```python
from build123d import *

# Parameters (mm, degrees)
F0_W     = 41.710345
F0_H     = 19.551726
F0_W_2   = 8.255173
F0_H_2   = 5.21379
F0_W_3   = 9.55862
F0_H_3   = 4.779309
F1_DEPTH = 25
F2_R     = 1.5
F3_R     = 0.55
F4_R     = 1
F5_SIZE  = 2


with BuildPart() as f1:
    # F0 (on Top) → F1 (new body)
    with BuildSketch(Plane.XY):
        with Locations((-29.001724, 36.931037)):
            Rectangle(F0_W, F0_H)
        with Locations((-38.343103, 34.975864)):
            Rectangle(F0_W_2, F0_H_2, mode=Mode.SUBTRACT)
        with Locations((-20.746552, 37.799999)):
            Rectangle(F0_W_3, F0_H_3, mode=Mode.SUBTRACT)
    extrude(amount=-F1_DEPTH)

    # F2
    f2_edges = [f1.edges().sort_by_distance(p)[0] for p in [
        (-42.47069, 37.582759, -12.5),
        (-34.215517, 37.582759, -12.5),
        (-42.47069, 32.368969, -12.5),
        (-34.215517, 32.368969, -12.5),
        (-25.525862, 40.189654, -12.5),
    ]]
    fillet(f2_edges, radius=F2_R)

    # F3
    f3_edges = [f1.edges().sort_by_distance(p)[0] for p in [
        (-15.967242, 40.189654, -12.5),
        (-25.525862, 35.410345, -12.5),
        (-15.967242, 35.410345, -12.5),
    ]]
    fillet(f3_edges, radius=F3_R)

    # F4
    f4_edges = [f1.edges().sort_by_distance(p)[0] for p in [
        (-38.343104, 37.582759, 0),
    ]]
    fillet(f4_edges, radius=F4_R)

    # F5
    f5_edges = [f1.edges().sort_by_distance(p)[0] for p in [
        (-20.271552, 40.189654, 0),
    ]]
    chamfer(f5_edges, length=F5_SIZE)


solid = f1.part
```
Source: CAD feature listing. Evaluate the final solid. Frame: model axes, mm. A direction names the side the tool comes from. Round coordinates to 2 decimals unless told otherwise and drop trailing zeros. Loops run counter-clockwise (first coordinate to the right, second up) from the corner with the lowest first, then second, coordinate; pieces in that order, holes last. Notation, with made-up numbers: M 30,3 L 42,3 A10 ccw 42,16 Z; hole C 43,28.25 d5. An arc over 180 degrees is marked long. Use a Markdown table: item, result. Add a question column.
1. Ray query, line 1 along Y through (x, z) = (-19, -10.5); line 2 along X through (y, z) = (35.75, -21.5); line 3 along X through (y, z) = (35.5, -21.5). Return the intervals inside material, ascending. Write a range as [from, to].
2. Cut plane A-A, the plane z = -18.75. Output: boundary loops of the cut face in (x, y), and give its area (3 significant figures).
3. Pull-direction query (Y, two-part tool) for faces 1 (the flat face through (-29, 46.707, -12)), 2 (the flat face through (-8.147, 37, -12)), 3 (the flat face through (-15.967, 38, -13)); classes: +Y half, -Y half, draft (parallel to the pull), parting line (faces both ways), or undercut.
4. Set-up query: faces 4 (the flat face through (-34.216, 35, -13)), 5 (the conical face through (-15.419, 34.886, -1.014)), 6 (the flat face through (-29, 27.155, -12)). Return all of +Z, -Z, +X, -X, +Y, -Y with unobstructed straight access to the full face (end or side cutting, diameter ignored); none if empty.
Solution:
| question | item | result |
|---|---|---|
| 1 | line 1 | y = [27.16, 35.41], [40.19, 46.71] |
| 1 | line 2 | x = [-49.86, -42.47], [-34.22, -25.48], [-16.01, -8.15] |
| 1 | line 3 | x = [-49.86, -42.47], [-34.22, -25.28], [-16.22, -8.15] |
| 2 | outline | M -49.86,27.16 L -8.15,27.16 L -8.15,46.71 L -49.86,46.71 Z; hole M -42.47,33.87 A1.5 ccw -40.97,32.37 L -35.72,32.37 A1.5 ccw -34.22,33.87 L -34.22,36.08 A1.5 ccw -35.72,37.58 L -40.97,37.58 A1.5 ccw -42.47,36.08 Z; hole M -25.53,35.96 A0.55 ccw -24.98,35.41 L -16.52,35.41 A0.55 ccw -15.97,35.96 L -15.97,39.64 A0.55 ccw -16.52,40.19 L -24.03,40.19 A1.5 ccw -25.53,38.69 Z |
| 2 | area | 729 mm2 |
| 3 | face 1 | +Y half |
| 3 | face 2 | draft |
| 3 | face 3 | undercut |
| 4 | face 4 | +Z, -Z |
| 4 | face 5 | +Z |
| 4 | face 6 | +Z, -Z, +X, -X, -Y |
